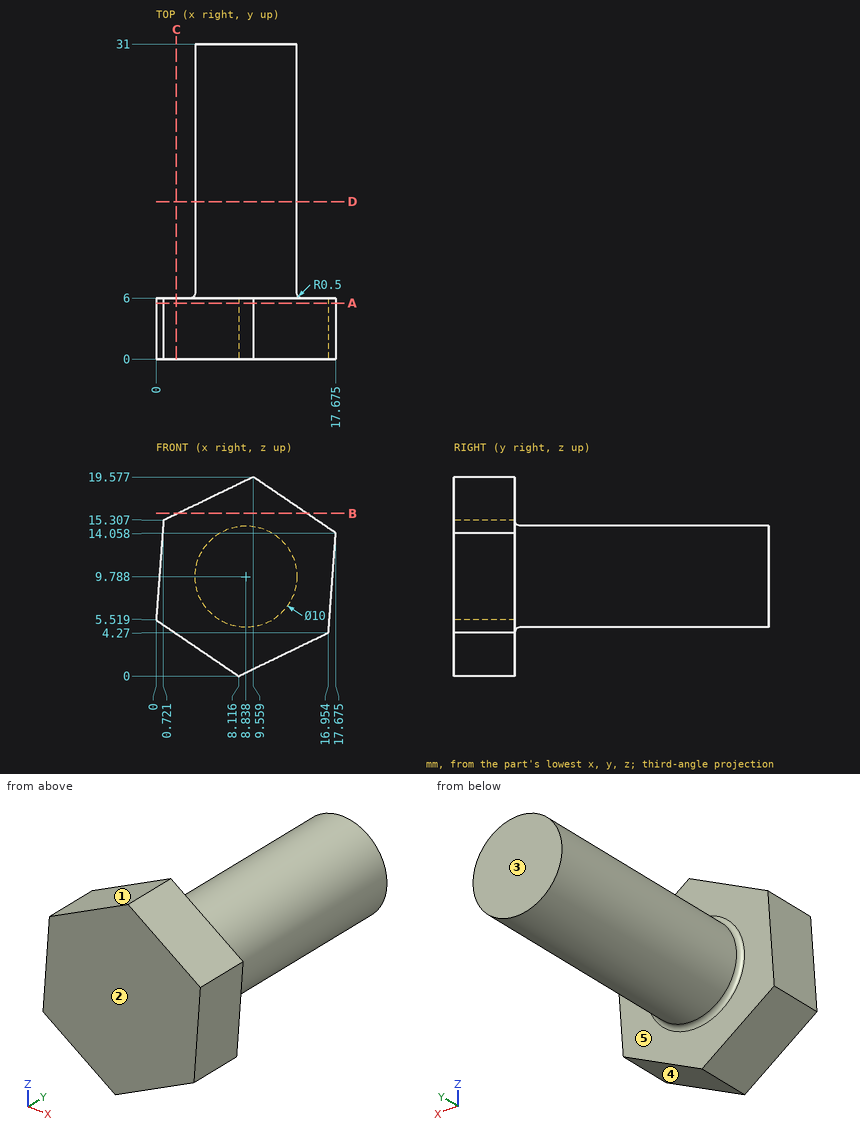
Job drawing, mm, ordinate dimensions from the low corner. One solid piece. A direction names the side the tool comes from. Coordinates: 2 decimals unless noted, no trailing zeros. Loops run counter-clockwise (first coordinate to the right, second up) from the corner with the lowest first, then second, coordinate; pieces in that order, holes last. Notation, with made-up numbers: (78.5, 39.25) - (120.5, 39.25) arc R33 ccw to (120.5, 73.25) - close; hole circle Ø4 at (-1.5, 77.5). An arc over 180 degrees is marked (long way). Write item = value, one per line. Start each with the question number.
Q1. Cut at B-B, the plane z = 16. List the corners of the cut face in (x, y) (1 decimal).
Q2. Pull direction Y, two halves, no side cores. Call the marked faces 1, 2 and 3: pulls with the +Y half, pulls with the -Y half, needs draft (parallel to the pull), parting line crosses it, or undercut.
Q3. Drill centre lines: L1, parallel to Y at x = 11.75, z = 18; L2, parallel to Z at x = 6.25, y = 7 (1 decimal); L3, parallel to X at y = 15.5, z = 10.25. Where is each one in solid material? Low to high.
Q4. Cut at D-D, the plane y = 15.5. List the corners of the cut face in (x, z).
Q5. Which spindle directions (+Z, -Z, +X, -X, +Y, -Y) get a long thin tool onto all of the face, cutting with end or side? Do the marked faces 4 and 5. Say none if no direction does.
Q6. Flat gauge pins, fed straight in: pin 1 Ø2 at (x, z) = (15, 11) entering from +Y; pin 2 Ø8 at (x, z) = (5, 12) entering from -Y; pin 3 Ø3 at (y, z) = (27.5, 11) entering from +X; pin 4 Ø6 at (y, z) = (13.5, 5.5) entering from -X. Where does each tip first touch, or does it go through?
Q7. Cut at C-C, the plane x = 2. List the corners of the cut face in (y, z) (1 decimal).
Q8. Cut at A-A, the plane y = 5.5. List the corners of the cut face in (x, z) (1 decimal).
Computed:
q1.outline = (2.2, 0) - (14.8, 0) - (14.8, 6) - (2.2, 6) - close
q2.face_1 = needs draft
q2.face_2 = pulls with the -Y half
q2.face_3 = pulls with the +Y half
q3.L1 = 0 to 6
q3.L2 = 5.5 to 14.1
q3.L3 = 3.86 to 13.82
q4.outline = circle Ø10 at (8.84, 9.79)
q5.face_4 = -Z, +X, +Y, -Y
q5.face_5 = +Y
q6.pin_1 = 6.05
q6.pin_2 = 0
q6.pin_3 = 13.84
q6.pin_4 = 4.01
q7.outline = (0, 4.2) - (6, 4.2) - (6, 15.9) - (0, 15.9) - close
q8.outline = (0, 5.5) - (8.1, 0) - (17, 4.3) - (17.7, 14.1) - (9.6, 19.6) - (0.7, 15.3) - close
